```python
from build123d import *

# Parameters (mm, degrees)
SKETCH2_R           = 2.1
SKETCH2_R_2         = 1.5
SKETCH2_W           = 40
SKETCH2_H           = 20
SKETCH2_W_2         = 10
SKETCH2_H_2         = 3
BOSS_EXTRUDE1_DEPTH = 3


with BuildPart() as part:
    # Sketch2 → Boss-Extrude1 (new body)
    with BuildSketch(Plane(origin=(0, 0, 0), x_dir=(1, 0, 0), z_dir=(0, 1, 0))):
        Polygon((0, 15.5), (9, 15.5), (9, 47.5), (-49, 47.5), (-49, 15.5), (-40, 15.5), (-40, 0), (-36, 0), (-36, -3), (-26, -3), (-26, 0), (-21.5, 0), (-21.5, 3.1), (-22.8, 3.1), (-22.8, 5.6), (-21.5, 5.6), (-21.5, 9.4), (-18.5, 9.4), (-18.5, 5.6), (-17.2, 5.6), (-17.2, 3.1), (-18.5, 3.1), (-18.5, 0), (-14, 0), (-14, -3), (-4, -3), (-4, 0), (0, 0), align=None)
        with Locations(Location((4.2, 25.5, 0), (0, 0, 270))):
            Circle(SKETCH2_R, mode=Mode.SUBTRACT)
        with Locations(Location((4.2, 37.3, 0), (0, 0, 270))):
            Circle(SKETCH2_R, mode=Mode.SUBTRACT)
        with Locations(Location((-44.2, 37.3, 0), (0, 0, 270))):
            Circle(SKETCH2_R, mode=Mode.SUBTRACT)
        with Locations(Location((-44.2, 25.5, 0), (0, 0, 270))):
            Circle(SKETCH2_R, mode=Mode.SUBTRACT)
        with Locations(Location((-20, 15.5, 0), (0, 0, 270))):
            Circle(SKETCH2_R_2, mode=Mode.SUBTRACT)
        with Locations((-20, 31.5)):
            Rectangle(SKETCH2_W, SKETCH2_H, mode=Mode.SUBTRACT)
        with Locations((-31, 15.5)):
            Rectangle(SKETCH2_W_2, SKETCH2_H_2, mode=Mode.SUBTRACT)
        with Locations((-9, 15.5)):
            Rectangle(SKETCH2_W_2, SKETCH2_H_2, mode=Mode.SUBTRACT)
    extrude(amount=BOSS_EXTRUDE1_DEPTH)


solid = part.part
```
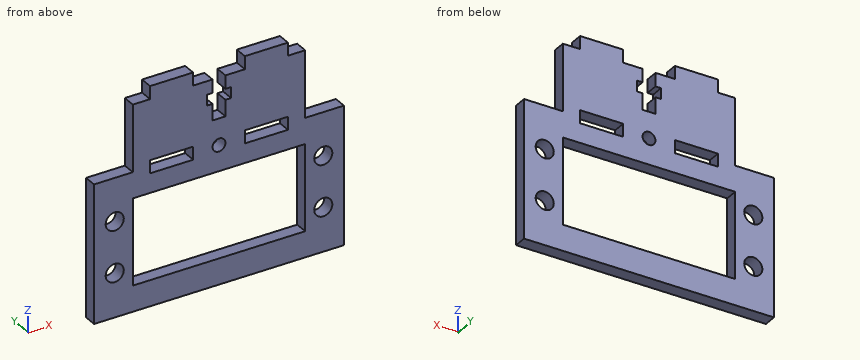
For this review, take the finished solid that the model builds, in its own axes (mm). Give positions to 0.01 mm unless a question says otherwise; leave off trailing zeros. Loops run counter-clockwise (first coordinate to the right, second up) from the corner with the lowest first, then second, coordinate; pieces in that order, holes last. Notation, with made-up numbers: M -20,-11 L -12,-11 A18 cw -12,19 Z; hole C 82,38 d5. An arc over 180 degrees is marked long. One line per item, written item: value. Start each with the question number.
Q1. Add section D-D (y = 2.3). Count the separate pieces of the cut face and the enclosed holes in it, and give its area (3 significant figures).
Q2. For L1, parallel to X at y = 1.3, z = -25.5; L2, parallel to Z at x = -27, y = 2.6; L3, parallel to X at y = 1, z = -30.5, list the stretches that pass through material, from the lowest coordinate up.
Q3. Clearance check with flat-ended pins moving along their axes: pin 1 Ø1.4 at (x, y) = (-18, 1) entering from +Z; pin 2 Ø1.5 at (x, y) = (6.5, 2) entering from +Z; pin 3 Ø1.5 at (y, z) = (1.5, -7) entering from -X. State where each tip first meets the part, or that it passes through.
Q4. Add section B-B (x = -32). Give the boundary of the cut face in (y, z), and give its area (3 significant figures).
Q5. Add section A-A (z = -37.3). Give the boundary of the cut face in (x, y), and give its area (3 significant figures).
Q6. Add section C-C (x = -38.5). Give the boundary of the cut face in (y, z), and give its area (3 significant figures).
Reply:
1. separate pieces: 1
1. enclosed holes: 8
1. area: 1,580 mm²
2. L1: -49 to -46.3, -42.1 to -40, 0 to 2.1, 6.3 to 9
2. L2: -47.5 to -41.5, -21.5 to -17, -14 to 3
2. L3: -49 to -40, 0 to 9
3. pin 1: z = 0
3. pin 2: z = -15.5
3. pin 3: x = -40
4. outline: M 0,-47.5 L 3,-47.5 L 3,-41.5 L 0,-41.5 Z; M 0,-21.5 L 3,-21.5 L 3,-17 L 0,-17 Z; M 0,-14 L 3,-14 L 3,3 L 0,3 Z
4. area: 82.5 mm²
5. outline: M -49,0 L -46.3,0 L -46.3,3 L -49,3 Z; M -42.1,0 L -40,0 L -40,3 L -42.1,3 Z; M 0,0 L 2.1,0 L 2.1,3 L 0,3 Z; M 6.3,0 L 9,0 L 9,3 L 6.3,3 Z
5. area: 28.8 mm²
6. outline: M 0,-47.5 L 3,-47.5 L 3,-41.5 L 0,-41.5 Z; M 0,-21.5 L 3,-21.5 L 3,0 L 0,0 Z
6. area: 82.5 mm²
